For this review, take the finished solid that the model builds, in its own axes (mm). A direction names the side the tool comes from. Coordinates: 2 decimals unless noted, no trailing zeros. Order: outer loops, then holes, each group sorted by start corner. A loop starts at its lowest first (then second) coordinate and runs counter-clockwise, first axis right, second up. Notation, with made-up numbers: (24.5, 23.25) -> (71.5, 23.25) arc R15 ccw to (71.5, 51.25) -> close; hole circle Ø6 at (18.5, 48.25). An arc over 180 degrees is marked (long way). Answer as a JSON object with one key per item and string values. Group by question number.
1) Wall thickness on L1, parallel to X at y = 3.5, z = 129; L2, parallel to X at y = 7.5, z = 146; L3, parallel to X at y = 3.75, z = 27.5: over which ranges is each line inside the solid? List them lowest first.
2) Add section B-B, the plane z = 118. Write out the cut boundary in (x, y), then the cut area to 3 significant figures.
3) For pin 1 (4 mm diameter, centred on y = 1, z = 66.5, fed in from +X); pin 2 (12 mm diameter, centred on x = 56, z = 43, fed in from +Y); pin 3 (4 mm diameter, centred on y = 2, z = 156, fed in from +X); pin 4 (5 mm diameter, centred on y = 3, z = 39, fed in from -X), all flat-tipped, find the tip position at first contact; note any pin that passes through.
4) Add section D-D, the plane x = 14.5. Write out the cut boundary in (y, z).
5) Draft analysis for pull direction X (two halves, no side actions). For faces 3 (the flat face through (14.23, 4.93, 141.54)), 4 (the flat face through (15.21, 4.93, 93.67)), 5 (the flat face through (55.21, 4.93, 96.33)), 6 (the flat face through (22, 10, 130)), state which applies: +X half, -X half, draft (parallel to the pull), parting line (faces both ways), or undercut.
6) Add section C-C, the plane x = 48.5. Write out the cut boundary in (y, z).
7) Add section A-A, the plane y = 4.25. Write out the cut boundary in (x, z).
8) Machinability: for faces 1 (the flat face through (35, 5, 0)), 2 (the flat face through (27.31, 4.93, 144.89)), which of the approach directions +Z, -Z, +X, -X, +Y, -Y give a long, thin tool a straight path to every point of the face, cutting with its end or side? Answer none if there is none.
from build123d import *

# Parameters (mm, degrees)
F0_W      = 80
F0_H      = 16
F1_DEPTH  = 160
F3_DEPTH  = 25
F5_DEPTH  = 25
F7_W      = 70
F7_H      = 10
F8_DEPTH  = 190
F10_DEPTH = 25
F12_DEPTH = 25
F14_DEPTH = 25
F16_DEPTH = 25


with BuildPart() as f1:
    # F0 (on Top) → F1 (new body)
    with BuildSketch(Plane.XY):
        with Locations((40, 8)):
            Rectangle(F0_W, F0_H)
    extrude(amount=F1_DEPTH)

    # F2 (on face) → F3 (cut)
    with BuildSketch(Plane.XZ):
        Polygon((0, 160), (0, 0), (32.5, 0), align=None)
    extrude(amount=-F3_DEPTH, mode=Mode.SUBTRACT)

    # F4 (on face) → F5 (cut)
    with BuildSketch(Plane.XZ):
        Polygon((47.5, 0), (80, 0), (80, 160), align=None)
    extrude(amount=-F5_DEPTH, mode=Mode.SUBTRACT)


with BuildPart() as f8:
    # F7 (on Top) → F8 (new body)
    with BuildSketch(Plane.XY):
        with Locations((35, 5)):
            Rectangle(F7_W, F7_H)
    extrude(amount=F8_DEPTH)

    # F9 (on face) → F10 (cut)
    with BuildSketch(Plane.XZ):
        Polygon((0, 190), (0, 0), (30, 0), align=None)
    extrude(amount=-F10_DEPTH, mode=Mode.SUBTRACT)

    # F11 (on face) → F12 (cut)
    with BuildSketch(Plane.XZ):
        Polygon((40, 0), (70, 0), (70, 190), align=None)
    extrude(amount=-F12_DEPTH, mode=Mode.SUBTRACT)

    # F13 (on face) → F14 (cut)
    with BuildSketch(Plane.XZ):
        Polygon((19.4037426527, 108.7762965329), (35, 10), (50.5962573473, 108.7762965329), (35, 180), align=None)
    extrude(amount=-F14_DEPTH, mode=Mode.SUBTRACT)

    # F15 (on face) → F16 (cut)
    with BuildSketch(Plane.XZ):
        Polygon((11.8801091279, 156.4259755233), (16.6473853285, 126.2332262527), (17.4916778251, 130.0888716859), (23.2588624734, 156.4259755233), (16.6473853285, 181.9978654385), align=None)
        Polygon((58.1198908721, 156.4259755233), (53.3526146715, 181.9978654385), (46.7411375266, 156.4259755233), (52.5083221749, 130.0888716859), (53.3526146715, 126.2332262527), align=None)
    extrude(amount=-F16_DEPTH, mode=Mode.SUBTRACT)


solid = f8.part
Output values:
{
 "1": {"L1": "x = 9.63 to 16.21, 17.25 to 23.83, 46.17 to 52.75, 53.79 to 60.37", "L2": "x = 6.95 to 13.53, 20.98 to 27.55, 42.45 to 49.02, 56.47 to 63.05", "L3": "x = 25.66 to 32.24, 37.76 to 44.34"},
 "2": {"outline": "(11.37, 0) -> (21.42, 0) -> (21.42, 10) -> (11.37, 10) -> close; (48.58, 0) -> (58.63, 0) -> (58.63, 10) -> (48.58, 10) -> close", "area": "201 mm²"},
 "3": {"pin 1": "stops at x = 50.82", "pin 2": "passes through", "pin 3": "stops at x = 64.95", "pin 4": "stops at x = 23.45"},
 "4": {"outline": "(0, 98.17) -> (10, 98.17) -> (10, 139.83) -> (0, 139.83) -> close; (0, 170.48) -> (10, 170.48) -> (10, 190) -> (0, 190) -> close"},
 "5": {"face 3": "undercut", "face 4": "-X half", "face 5": "+X half", "face 6": "draft"},
 "6": {"outline": "(0, 53.83) -> (10, 53.83) -> (10, 95.5) -> (0, 95.5) -> close; (0, 118.35) -> (10, 118.35) -> (10, 148.39) -> (0, 148.39) -> close; (0, 163.23) -> (10, 163.23) -> (10, 190) -> (0, 190) -> close"},
 "7": {"outline": "(0, 190) -> (30, 0) -> (40, 0) -> (70, 190) -> close; hole (11.88, 156.43) -> (16.65, 126.23) -> (23.26, 156.43) -> (16.65, 182) -> close; hole (19.4, 108.78) -> (35, 10) -> (50.6, 108.78) -> (35, 180) -> close; hole (46.74, 156.43) -> (53.35, 126.23) -> (58.12, 156.43) -> (53.35, 182) -> close"},
 "8": {"face 1": "-Z, +X, -X, +Y, -Y", "face 2": "+Y, -Y"}
}
